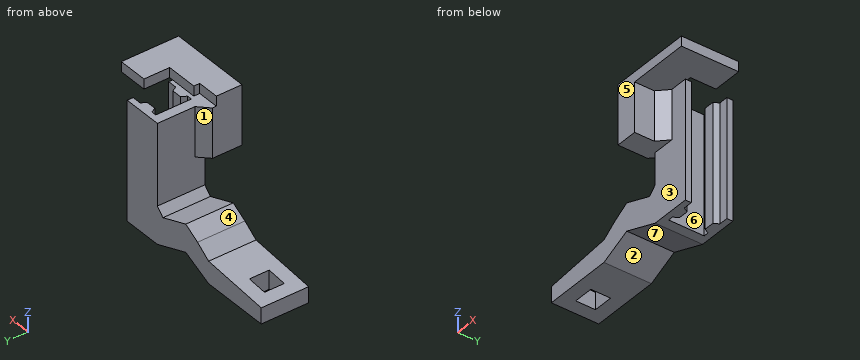
from build123d import *

# Parameters (mm, degrees)
BOSS_EXTRUDE1_DEPTH = 30
SKETCH2_W           = 11
SKETCH2_H           = 25
BOSS_EXTRUDE2_DEPTH = 15
CHAMFER1_SIZE       = 5
SKETCH3_W           = 42
SKETCH3_H           = 13
BOSS_EXTRUDE3_DEPTH = 5
BOSS_EXTRUDE4_DEPTH = 5
BOSS_EXTRUDE5_DEPTH = 24
CHAMFER2_SIZE       = 5
CHAMFER2_SIZE2      = 3.901030044
BOSS_EXTRUDE6_DEPTH = 24
SKETCH7_W           = 10
SKETCH7_H           = 10
CUT_EXTRUDE1_DEPTH  = 10


with BuildPart() as part:
    # Sketch1 → Boss-Extrude1 (new, symmetric)
    with BuildSketch(Plane.XY.offset(-109.087000354)):
        Polygon((-916.669839571, 150.370500968), (-916.669839571, 153.370500968), (-936.669839571, 153.370500968), (-936.669839571, 129.370500968), (-916.669839571, 129.370500968), (-916.669839571, 132.370500968), (-921.283088225, 132.370500968), (-922.726463898, 134.870500968), (-927.726463898, 134.870500968), (-929.169839571, 132.370500968), (-931.669839571, 132.370500968), (-931.669839571, 150.370500968), (-929.169839571, 150.370500968), (-927.726463898, 147.870500968), (-922.726463898, 147.870500968), (-921.283088225, 150.370500968), align=None)
    extrude(amount=BOSS_EXTRUDE1_DEPTH, both=True)

    # Sketch2 → Boss-Extrude2 (add)
    with BuildSketch(Plane.XZ.offset(-129.370500968)):
        with Locations((-936.169839571, -91.587000354)):
            Rectangle(SKETCH2_W, SKETCH2_H)
    extrude(amount=BOSS_EXTRUDE2_DEPTH)

    # Chamfer1
    chamfer1_edges = [part.edges().sort_by_distance(p)[0] for p in [
        (-936.669839571, 129.370500968, -91.587000354),
        (-930.669839571, 129.370500968, -91.587000354),
    ]]
    chamfer(chamfer1_edges, length=CHAMFER1_SIZE - 0.0001)  # a hair under: the kernel refuses the full size

    # Sketch3 → Boss-Extrude3 (add)
    with BuildSketch(Plane.XY.offset(-79.087000354)):
        with Locations((-920.669839571, 120.870500968)):
            Rectangle(SKETCH3_W, SKETCH3_H)
    extrude(amount=BOSS_EXTRUDE3_DEPTH)

    # Sketch4 → Boss-Extrude4 (add)
    with BuildSketch(Plane.XY.offset(-74.087000354)):
        Polygon((-899.669839571, 127.370500968), (-899.669839571, 143.370500968), (-914.669839571, 143.370500968), (-914.669839571, 130.370500968), (-930.669839571, 130.370500968), (-930.669839571, 127.370500968), align=None)
    extrude(amount=-BOSS_EXTRUDE4_DEPTH)

    # Sketch5 → Boss-Extrude5 (add)
    with BuildSketch(Plane(origin=(0, 153.370500968, 0), x_dir=(1, 0, 0), z_dir=(0, 1, 0))):
        Polygon((-936.669839571, 139.087000354), (-936.669839571, 125.087000354), (-955.463691986, 118.246597487), (-955.463691986, 132.246597487), align=None)
    extrude(amount=-BOSS_EXTRUDE5_DEPTH)

    # Chamfer2
    chamfer2_edges = [part.edges().sort_by_distance(p)[0] for p in [
        (-936.669839571, 141.370500968, -125.087000354),
    ]]
    chamfer2_side = [part.faces().sort_by_distance(p)[0] for p in [
        (-936.669839571, 142.583452416, -103.427623846),
    ]]
    chamfer(chamfer2_edges, length=CHAMFER2_SIZE, length2=CHAMFER2_SIZE2, reference=chamfer2_side[0])

    # Sketch6 → Boss-Extrude6 (add)
    with BuildSketch(Plane(origin=(0, 153.370500968, 0), x_dir=(1, 0, 0), z_dir=(0, 1, 0))):
        Polygon((-955.463691986, 132.246597487), (-970.605038874, 139.087000354), (-1005.463691986, 139.087000354), (-1005.463691986, 131.087000354), (-970.605038874, 127.94465995), (-963.25792062, 122.746597487), (-955.463691986, 118.246597487), align=None)
    extrude(amount=-BOSS_EXTRUDE6_DEPTH)

    # Sketch7 → Cut-Extrude1 (cut)
    with BuildSketch(Plane(origin=(0, 0, -139.087000354), x_dir=(-1, 0, 0), z_dir=(0, 0, -1))):
        with Locations((993.463691986, 141.370500968)):
            Rectangle(SKETCH7_W, SKETCH7_H)
    extrude(amount=-CUT_EXTRUDE1_DEPTH, mode=Mode.SUBTRACT)


solid = part.part
Can you work these out from the model? Positions are in its coordinate system, mm. Face numbers are marked on the shaded views. A direction names the side the tool comes from. Coordinates: 2 decimals unless noted, no trailing zeros. Order: outer loops, then holes, each group sorted by start corner. A loop starts at its lowest first (then second) coordinate and runs counter-clockwise, first axis right, second up. Notation, with made-up numbers: M 59.25,26 L 102.25,26 A18 ccw 102.25,57 Z; hole C 58,75 d3. An arc over 180 degrees is marked long. Write item = value, one per line.
(1) Suppose I cut it at A-A on x = -924.5. Please give me the cut outline in (y, z).
Results are:
outline = M 114.37,-79.09 L 129.37,-79.09 L 129.37,-139.09 L 134.87,-139.09 L 134.87,-79.09 L 130.37,-79.09 L 130.37,-74.09 L 114.37,-74.09 Z; M 147.87,-139.09 L 153.37,-139.09 L 153.37,-79.09 L 147.87,-79.09 Z
(2) Suppose I cut it at B-B on y = 138. Please give me the cut outline in (x, z).
Results are:
outline = M -1005.46,-139.09 L -998.46,-139.09 L -998.46,-130.46 L -1005.46,-131.09 Z; M -988.46,-139.09 L -970.61,-139.09 L -955.46,-132.25 L -936.67,-139.09 L -931.67,-139.09 L -931.67,-79.09 L -936.67,-79.09 L -936.67,-120.09 L -940.34,-123.75 L -955.46,-118.25 L -963.26,-122.75 L -970.61,-127.94 L -988.46,-129.55 Z; M -914.67,-79.09 L -899.67,-79.09 L -899.67,-74.09 L -914.67,-74.09 Z
(3) Suppose I cut it at D-D on y = 118. Please give me the cut outline in (x, z), plus the area to 3 significant figures.
Results are:
outline = M -941.67,-104.09 L -930.67,-104.09 L -930.67,-79.09 L -899.67,-79.09 L -899.67,-74.09 L -941.67,-74.09 Z
area = 485 mm2
(4) I need wall thicknesses on line 1 along X through (y, z) = (133, -77); line 2 along Y through (x, z) = (-920, -82.5); line 3 along Z through (x, y) = (-920, 127.5). Which ranges of each line are inside material? Lowest first, please. Write a range as [from, to].
Results are:
line_1 = [-914.67, -899.67]
line_2 = [129.37, 132.37], [150.37, 153.37]
line_3 = [-79.09, -74.09]
(5) For the marked faces 1, 2 and 3, which set-ups out of +Z, -Z, +X, -X, +Y, -Y let a thin tool reach every point of the face, with its end or its side?
Results are:
face_1 = +Z, -X, +Y
face_2 = -Z, +Y, -Y
face_3 = -Z, +X, -Y
(6) If we mould it in two halves opening along X, with no side actions, what happens to the marked faces 4, 5, 6 and 7? For each: pulls with the +X half, pulls with the -X half, needs draft (parallel to the pull), parting line crosses it, or undercut.
Results are:
face_4 = pulls with the -X half
face_5 = needs draft
face_6 = undercut
face_7 = undercut
(7) For pin 1 Ø8 at (x, z) = (-968, -118.5) entering from -Y; pin 2 Ø3 at (x, y) = (-967.5, 139.5) entering from -Z; pin 3 Ø5 at (x, y) = (-934, 132.5) entering from +Z; pin 4 Ø1.5 at (y, z) = (151.5, -110) entering from +X, each with a flat end and sliding along its axis, tell me the tip position at first contact or that it passes through.
Results are:
pin_1 = through
pin_2 = -138.36
pin_3 = -79.09
pin_4 = -916.67
